CAD build for the part. Positions are in the model's coordinates, mm. A direction names the side the tool comes from. Coordinates: 2 decimals unless noted, no trailing zeros. Loops run counter-clockwise (first coordinate to the right, second up) from the corner with the lowest first, then second, coordinate; pieces in that order, holes last.
1) Pin check, flat tips, straight feed: pin 1 Ø1.1 at (y, z) = (0, -4) entering from +X; pin 2 Ø1.1 at (y, z) = (0, -5) entering from -X; pin 3 Ø1 at (y, z) = (1.5, 16) entering from +X. Stop position of each tip, or through.
2) Saw through at C-C, the plane z = 35. Write the cut outline in (x, y).
3) Saw through at B-B, the plane y = -3.25. Write the cut outline in (x, z), and give its area (3 significant figures).
4) Which spindle directions (+Z, -Z, +X, -X, +Y, -Y) get a long thin tool onto all of the face, cutting with end or side? Do faces 1 (the flat face through (8, 5.5, -3)), 2 (the cylindrical face through (20, -4.07, -3.45)), 3 (the cylindrical face through (-5.07, -4, -3.45)), 4 (the flat face through (7, -5.5, -3)). Say none if no direction does.
5) Wall check: line 1 along Z through (x, y) = (21.25, -2.5); line 2 along X through (y, z) = (-3.75, 37.5); line 3 along Y through (x, z) = (3.25, -3.5). Give the ranges that are in metal, low to high.
6) Saw through at A-A, the plane x = 12.5. Write the cut outline in (y, z).
```python
from build123d import *

# Parameters (mm, degrees)
BOSS_EXTRUDE1_DEPTH = 57
BOSS_EXTRUDE2_DEPTH = 7


with BuildPart() as part:
    # Sketch1 → Boss-Extrude1 (new body)
    with BuildSketch(Plane.XY):
        with BuildLine():
            Line((0, 7.5), (15, 7.5))
            ThreePointArc((15, 7.5), (22.5, 0), (15, -7.5))
            Line((15, -7.5), (0, -7.5))
            ThreePointArc((0, -7.5), (-7.5, 0), (0, 7.5))
        make_face()
    extrude(amount=BOSS_EXTRUDE1_DEPTH)

    # Sketch3 → Boss-Extrude2 (add)
    with BuildSketch(Plane(origin=(0, 0, 0), x_dir=(-1, 0, 0), z_dir=(0, 0, -1))):
        with BuildLine():
            Line((-16.5, 5.5), (1.5, 5.5))
            ThreePointArc((1.5, 5.5), (5.035533906, 4.035533906), (6.5, 0.5))
            Line((6.5, 0.5), (6.5, -0.5))
            ThreePointArc((6.5, -0.5), (5.035533906, -4.035533906), (1.5, -5.5))
            Line((1.5, -5.5), (-16.5, -5.5))
            ThreePointArc((-16.5, -5.5), (-20.035533906, -4.035533906), (-21.5, -0.5))
            Line((-21.5, -0.5), (-21.5, 0.5))
            ThreePointArc((-21.5, 0.5), (-20.035533906, 4.035533906), (-16.5, 5.5))
        make_face()
    extrude(amount=BOSS_EXTRUDE2_DEPTH)


solid = part.part
```
Data:
1. pin 1: stops at x = 21.5
1. pin 2: stops at x = -6.5
1. pin 3: stops at x = 22.43
2. outline: (0, -7.5) - (15, -7.5) arc R7.5 ccw to (15, 7.5) - (0, 7.5) arc R7.5 ccw to start
3. outline: (-6.76, 0) - (-5.68, 0) - (-5.68, -7) - (20.68, -7) - (20.68, 0) - (21.76, 0) - (21.76, 57) - (-6.76, 57) - close
3. area: 1,810 mm2
4. face 1: -Z, +X, -X, +Y
4. face 2: -Z, +X, -Y
4. face 3: -Z, -X, -Y
4. face 4: -Z, +X, -X, -Y
5. line 1: z = 0 to 57
5. line 2: x = -6.5 to 21.5
5. line 3: y = -5.5 to 5.5
6. outline: (-7.5, 0) - (-5.5, 0) - (-5.5, -7) - (5.5, -7) - (5.5, 0) - (7.5, 0) - (7.5, 57) - (-7.5, 57) - close
